```python
from build123d import *

# Parameters (mm, degrees)
SKETCH2_R           = 76
BOSS_EXTRUDE1_DEPTH = 17.78
CUT_EXTRUDE3_DEPTH  = 6.604
CUT_EXTRUDE5_DEPTH  = 1.27
SKETCH10_W          = 41.91
SKETCH10_H          = 10.16
CUT_EXTRUDE6_DEPTH  = 1.016
SKETCH11_W          = 44.45
SKETCH11_H          = 44.45
BOSS_EXTRUDE2_DEPTH = 1.27
SKETCH14_R          = 3.175
BOSS_EXTRUDE4_DEPTH = 5.08
SKETCH15_R          = 73.66
BOSS_EXTRUDE5_DEPTH = 2.54
SKETCH16_R          = 3.175
CUT_EXTRUDE8_DEPTH  = 12.7


with BuildPart() as part:
    # Sketch2 → Boss-Extrude1 (new body)
    with BuildSketch(Plane(origin=(0, 0, 0), x_dir=(1, 0, 0), z_dir=(0, 1, 0))):
        Circle(SKETCH2_R)
    extrude(amount=BOSS_EXTRUDE1_DEPTH)

    # Sketch6 → Cut-Extrude3 (cut)
    with BuildSketch(Plane(origin=(0, 17.78, 0), x_dir=(1, 0, 0), z_dir=(0, 1, 0))):
        with BuildLine():
            Line((-76, 54.61), (76, 54.61))
            ThreePointArc((76, 54.61), (130.61, 0), (76, -54.61))
            Line((76, -54.61), (-76, -54.61))
            ThreePointArc((-76, -54.61), (-130.61, 0), (-76, 54.61))
        make_face()
    extrude(amount=-CUT_EXTRUDE3_DEPTH, mode=Mode.SUBTRACT)

    # Sketch9 → Cut-Extrude5 (cut)
    with BuildSketch(Plane(origin=(0, 11.176, 0), x_dir=(1, 0, 0), z_dir=(0, 1, 0))):
        with BuildLine():
            Line((-76, 25.4), (-25.4, 25.4))
            Line((-25.4, 25.4), (25.4, 25.4))
            Line((25.4, 25.4), (76, 25.4))
            ThreePointArc((76, 25.4), (101.4, 0), (76, -25.4))
            Line((76, -25.4), (25.4, -25.4))
            Line((25.4, -25.4), (-25.4, -25.4))
            Line((-25.4, -25.4), (-76, -25.4))
            ThreePointArc((-76, -25.4), (-101.4, 0), (-76, 25.4))
        make_face()
    extrude(amount=-CUT_EXTRUDE5_DEPTH, mode=Mode.SUBTRACT)

    # Sketch10 → Cut-Extrude6 (cut)
    with BuildSketch(Plane(origin=(0, 9.906, 0), x_dir=(1, 0, 0), z_dir=(0, 1, 0))):
        with Locations((-48.79885899, 13.97)):
            Rectangle(SKETCH10_W, SKETCH10_H)
        with Locations((-48.79885899, -13.97)):
            Rectangle(SKETCH10_W, SKETCH10_H)
        with Locations((48.79885899, -13.97)):
            Rectangle(SKETCH10_W, SKETCH10_H)
        with Locations((48.79885899, 13.97)):
            Rectangle(SKETCH10_W, SKETCH10_H)
    extrude(amount=-CUT_EXTRUDE6_DEPTH, mode=Mode.SUBTRACT)

    # Sketch11 → Boss-Extrude2 (add)
    with BuildSketch(Plane(origin=(0, 9.906, 0), x_dir=(1, 0, 0), z_dir=(0, 1, 0))):
        Rectangle(SKETCH11_W, SKETCH11_H)
    extrude(amount=BOSS_EXTRUDE2_DEPTH)

    # Sketch14 → Boss-Extrude4 (add)
    with BuildSketch(Plane(origin=(0, 11.176, 0), x_dir=(1, 0, 0), z_dir=(0, 1, 0))):
        Circle(SKETCH14_R)
    extrude(amount=BOSS_EXTRUDE4_DEPTH)

    # Sketch15 → Boss-Extrude5 (add)
    with BuildSketch(Plane.XZ):
        Circle(SKETCH15_R)
    extrude(amount=BOSS_EXTRUDE5_DEPTH)

    # Sketch16 → Cut-Extrude8 (cut)
    with BuildSketch(Plane.XZ.offset(2.54)):
        with Locations((0, 64.77)):
            Circle(SKETCH16_R)
        with Locations((0, -64.77)):
            Circle(SKETCH16_R)
    extrude(amount=-CUT_EXTRUDE8_DEPTH, mode=Mode.SUBTRACT)


solid = part.part
```
The listing builds one solid part. Answer for the finished solid, in the listing's coordinates (mm). A direction names the side the tool comes from. Give positions to 0.01 mm unless a question says otherwise; leave off trailing zeros. Loops run counter-clockwise (first coordinate to the right, second up) from the corner with the lowest first, then second, coordinate; pieces in that order, holes last. Notation, with made-up numbers: (54.5, 73) - (113.5, 73) arc R32 ccw to (113.5, 109) - close; hole circle Ø8 at (-39, -31). An arc over 180 degrees is marked (long way). Return JSON: item names as keys, results as strings. Group by question number.
1. Find section C-C (y = 2.5). Write down the section's boundary in (x, z) (3 decimals), then the cut area to 3 significant figures.
2. Find section D-D (z = -35). Write down the section's boundary in (x, y), then the cut area to 3 significant figures.
3. Determine the mould class of faces 6 (the flat face through (1, 9.906, -23)), 7 (the cylindrical face through (-58.454, -1.252, -44.821)), 8 (the cylindrical face through (1.707, 3.721, -62.093)) for opening direction X: pulls with the +X half, pulls with the -X half, needs draft (parallel to the pull), parting line crosses it, or undercut.
4. Straight lines are drawn through the part: line 1 (Z direction, x = 0, y = 0.25) (3 decimals); line 2 (Y direction, x = -33.5, z = -50.5); line 3 (Y direction, x = -28.5, z = -22.5). For each, find the intervals that lie inside material, in ascending order. Write a range as [from, to].
5. Given pin 1 Ø0.8 at (y, z) = (9.5, 12.5) entering from -X; pin 2 Ø15 at (x, z) = (-30.5, 4) entering from +Y; pin 3 Ø1.4 at (x, y) = (-35, 10.5) entering from +Z, each flat-ended and moving along its own axis, determine where each tip first touches the part or whether it passes through.
6. Find section B-B (z = 0). Write down the section's boundary in (x, y) (3 decimals), then the cut area to 3 significant figures.
7. Which of the six approach directions +Z, -Z, +X, -X, +Y, -Y give full straight-line access (tool end or side, diameter ignored) to faces 1 (the flat face through (-1, 17.78, -63)), 2 (the flat face through (0, 10.16, -65)), 3 (the flat face through (-49, 8.89, 14)), 4 (the cylindrical face through (70.205, 6.79, 29.108)), 5 (the flat face through (1, 15, 54.61))?
Verdict:
{
 "1": {"outline": "circle Ø152 at (0, 0); hole circle Ø6.35 at (0, -64.77); hole circle Ø6.35 at (0, 64.77)", "area": "18,100 mm^2"},
 "2": {"outline": "(-67.46, 0) - (-64.81, 0) - (-64.81, -2.54) - (64.81, -2.54) - (64.81, 0) - (67.46, 0) - (67.46, 11.18) - (-67.46, 11.18) - close", "area": "1,840 mm^2"},
 "3": {"face 6": "needs draft", "face 7": "parting line crosses it", "face 8": "undercut"},
 "4": {"line 1": "z = [-76, -67.945], [-61.595, 61.595], [67.945, 76]", "line 2": "y = [-2.54, 11.18]", "line 3": "y = [-2.54, 9.91]"},
 "5": {"pin 1": "stops at x = -75.03", "pin 2": "stops at y = 9.91", "pin 3": "stops at z = 67.82"},
 "6": {"outline": "(-76, 0) - (-73.66, 0) - (-73.66, -2.54) - (73.66, -2.54) - (73.66, 0) - (76, 0) - (76, 9.906) - (22.225, 9.906) - (22.225, 11.176) - (3.175, 11.176) - (3.175, 16.256) - (-3.175, 16.256) - (-3.175, 11.176) - (-22.225, 11.176) - (-22.225, 9.906) - (-76, 9.906) - close", "area": "1,970 mm^2"},
 "7": {"face 1": "+Z, -Z, +X, -X, +Y", "face 2": "-Y", "face 3": "+Y", "face 4": "+Y, -Y", "face 5": "+X, -X, +Y"}
}
